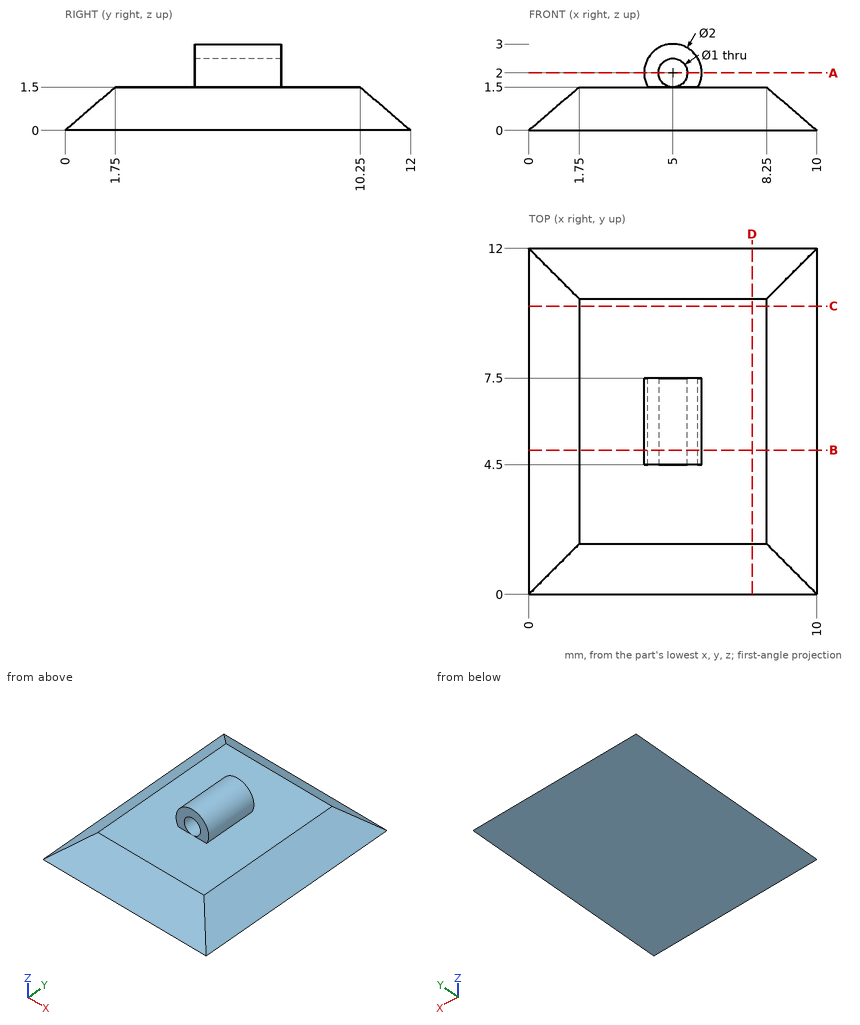
Can you work these out from the drawing? Everything is in mm from the part's minimum corner. Give positions to 0.01 mm unless a question says otherwise; leave off trailing zeros. Loops run counter-clockwise (first coordinate to the right, second up) from the corner with the lowest first, then second, coordinate; pieces in that order, holes last. Notation, with made-up numbers: M -38,-31 L 6,-31 A10 ccw 6,-17 Z; hole C -26,-9 d7. An arc over 180 degrees is marked long. Use CSV: the item, a comma, the result in double quotes. Start each with the question number.
1. If I drill on L1, parallel to X at y = 5.15, z = 2; L2, parallel to Z at x = 2.25, y = 10; L3, parallel to Y at x = 2.75, z = 0.25, over which ranges is the centre line in solid material (lowest first)?
2. For P1, Ø1.2, axis at x = 5, z = 2, coming from the -Y side; P2, Ø1.5, axis at x = 3, z = 2, coming from the +Y side; P3, Ø1.2, axis at x = 4.5, z = 2.5, coming from the +Y side, each with a flat end and sliding along its axis, tell me the tip position at first contact or that it passes through.
3. Imagine slicing it at A-A, the plane z = 2. Write out the boundary of the cut face in (x, y).
4. Imagine slicing it at D-D, the plane x = 7.75. Write out the boundary of the cut face in (y, z), plus the area to 3 significant figures.
5. Imagine slicing it at B-B, the plane y = 5. Write out the boundary of the cut face in (x, z).
6. Imagine slicing it at C-C, the plane y = 10. Write out the boundary of the cut face in (x, z).
Response values:
1,L1,"4 to 4.5, 5.5 to 6"
1,L2,"0 to 1.5"
1,L3,"0.29 to 11.71"
2,P1,"y = 1.63"
2,P2,"y = 10.54"
2,P3,"y = 7.5"
3,outline,"M 4,4.5 L 4.5,4.5 L 4.5,7.5 L 4,7.5 Z; M 5.5,4.5 L 6,4.5 L 6,7.5 L 5.5,7.5 Z"
4,outline,"M 0,0 L 12,0 L 10.25,1.5 L 1.75,1.5 Z"
4,area,"15.4 mm^2"
5,outline,"M 0,0 L 10,0 L 8.25,1.5 L 5.87,1.5 A1 ccw long 4.13,1.5 L 1.75,1.5 Z; hole C 5,2 d1"
6,outline,"M 0,0 L 10,0 L 8.25,1.5 L 1.75,1.5 Z"
